from build123d import *

# Parameters (mm, degrees)
SKETCH1_W                                     = 38.1
SKETCH1_H                                     = 44.45
BOSS_EXTRUDE1_DEPTH                           = 5
SKETCH2_W                                     = 38.1
SKETCH2_H                                     = 5
BOSS_EXTRUDE2_DEPTH                           = 25.4
CSK_FOR_8_FLAT_HEAD_SOCKET_CAP_SCREW1_A_COUNT = 2
CSK_FOR_8_FLAT_HEAD_SOCKET_CAP_SCREW1_A_PITCH = 12.7
CSK_FOR_8_FLAT_HEAD_SOCKET_CAP_SCRE_2_COUNT   = 2
CSK_FOR_8_FLAT_HEAD_SOCKET_CAP_SCRE_2_PITCH   = 27.043545921
CSK_FOR_8_FLAT_HEAD_SOCKET_CAP_SCRE_3_COUNT   = 2
CSK_FOR_8_FLAT_HEAD_SOCKET_CAP_SCRE_3_PITCH   = 23.876
CSK_FOR_8_FLAT_HEAD_SOCKET_CAP_SCREW2_A_COUNT = 2
CSK_FOR_8_FLAT_HEAD_SOCKET_CAP_SCREW2_A_PITCH = 19.05
FILLET1_R                                     = 5.08
FILLET2_R                                     = 5.08
FILLET3_R                                     = 1.27


with BuildPart() as part:
    # Sketch1 → Boss-Extrude1 (new body)
    with BuildSketch(Plane.XY):
        with Locations((19.05, 22.225)):
            Rectangle(SKETCH1_W, SKETCH1_H)
    extrude(amount=BOSS_EXTRUDE1_DEPTH)

    # Sketch2 → Boss-Extrude2 (add)
    with BuildSketch(Plane(origin=(0, 0, 0), x_dir=(-1, 0, 0), z_dir=(0, 0, -1))):
        with Locations((-19.05, 2.5)):
            Rectangle(SKETCH2_W, SKETCH2_H)
    extrude(amount=BOSS_EXTRUDE2_DEPTH)

    # Sketch4 → CSK for #8 Flat Head Socket Cap Screw1 (revolve, cut)
    with BuildSketch(Plane(origin=(25.4, 38.1, 0), x_dir=(0, 1, 0), z_dir=(1, 0, 0))):
        Polygon((0, 0), (0, 5), (2.2479, 5), (2.2479, 2.658961536), (4.5593, 0), align=None)
    csk_for_8_flat_head_socket_cap_screw1 = revolve(axis=Axis((25.4, 38.1, -6.35), (0, 0, 1)), mode=Mode.SUBTRACT)

    # CSK for #8 Flat Head Socket Cap Screw1 a: CSK for #8 Flat Head Socket Cap Screw1 ×2
    with Locations(*[(-i * CSK_FOR_8_FLAT_HEAD_SOCKET_CAP_SCREW1_A_PITCH, 0, 0) for i in range(1, CSK_FOR_8_FLAT_HEAD_SOCKET_CAP_SCREW1_A_COUNT)]):
        add(csk_for_8_flat_head_socket_cap_screw1, mode=Mode.SUBTRACT)

    # CSK for _8 Flat Head Socket Cap Scre 2: CSK for #8 Flat Head Socket Cap Screw1 ×2
    with Locations(*[Vector(-0.4696129729783402, -0.8828723891992799, 0) * (i * CSK_FOR_8_FLAT_HEAD_SOCKET_CAP_SCRE_2_PITCH) for i in range(1, CSK_FOR_8_FLAT_HEAD_SOCKET_CAP_SCRE_2_COUNT)]):
        add(csk_for_8_flat_head_socket_cap_screw1, mode=Mode.SUBTRACT)

    # CSK for _8 Flat Head Socket Cap Scre 3: CSK for #8 Flat Head Socket Cap Screw1 ×2
    with Locations(*[(0, -i * CSK_FOR_8_FLAT_HEAD_SOCKET_CAP_SCRE_3_PITCH, 0) for i in range(1, CSK_FOR_8_FLAT_HEAD_SOCKET_CAP_SCRE_3_COUNT)]):
        add(csk_for_8_flat_head_socket_cap_screw1, mode=Mode.SUBTRACT)

    # Sketch6 → CSK for #8 Flat Head Socket Cap Screw2 (revolve, cut)
    with BuildSketch(Plane(origin=(28.575, 5, -12.7), x_dir=(0, 0, 1), z_dir=(1, 0, 0))):
        Polygon((0, 0), (0, 5), (2.2479, 5), (2.2479, 2.658961536), (4.5593, 0), align=None)
    csk_for_8_flat_head_socket_cap_screw2 = revolve(axis=Axis((28.575, 11.35, -12.7), (0, -1, 0)), mode=Mode.SUBTRACT)

    # CSK for #8 Flat Head Socket Cap Screw2 a: CSK for #8 Flat Head Socket Cap Screw2 ×2
    with Locations(*[(-i * CSK_FOR_8_FLAT_HEAD_SOCKET_CAP_SCREW2_A_PITCH, 0, 0) for i in range(1, CSK_FOR_8_FLAT_HEAD_SOCKET_CAP_SCREW2_A_COUNT)]):
        add(csk_for_8_flat_head_socket_cap_screw2, mode=Mode.SUBTRACT)

    # Fillet1
    fillet1_edges = [part.edges().sort_by_distance(p)[0] for p in [
        (19.05, 5, 0),
    ]]
    fillet(fillet1_edges, radius=FILLET1_R)

    # Fillet2
    fillet2_edges = [part.edges().sort_by_distance(p)[0] for p in [
        (19.05, 0, 5),
    ]]
    fillet(fillet2_edges, radius=FILLET2_R)

    # Fillet3
    fillet3_edges = [part.edges().sort_by_distance(p)[0] for p in [
        (38.1, 24.765, 5),
        (38.1, 0, -12.74),
        (38.1, 1.487897552, 3.512102448),
        (0, 0, -12.74),
        (0, 1.487897552, 3.512102448),
        (38.1, 5, -15.24),
        (0, 5, -15.24),
        (38.1, 2.5, -25.4),
        (19.05, 44.45, 5),
        (19.05, 0, -25.4),
        (0, 2.5, -25.4),
        (19.05, 5, -25.4),
        (0, 24.765, 5),
        (19.05, 44.45, 0),
        (0, 27.265, 0),
        (38.1, 27.265, 0),
        (38.1, 6.487897552, -1.487897552),
        (0, 44.45, 2.5),
        (0, 6.487897552, -1.487897552),
        (38.1, 44.45, 2.5),
    ]]
    fillet(fillet3_edges, radius=FILLET3_R)


solid = part.part
Check sheet for the modelled part. Datum: model origin and axes. Units: mm. A direction names the side the tool comes from. Give positions to 0.01 mm unless a question says otherwise; leave off trailing zeros. Write each loop counter-clockwise with the first axis right and the second up, starting at its lowest first coordinate (ties: lowest second). Pieces come first, ordered by that corner, then holes. Notation, with made-up numbers: (2, 68.25) -> (15, 68.25) arc R21 cw to (15, 91.25) -> close; hole circle Ø2 at (-17.5, 76.25). An arc over 180 degrees is marked (long way). One line per item, written item: value. Start each with the question number.
Item 1: Gauge pin test, flat ends, axial feed: pin 1 (10 mm diameter, centred on x = 19.5, y = 28.5, fed in from -Z); pin 2 (4 mm diameter, centred on x = 12.7, y = 38.1, fed in from -Z); pin 3 (5 mm diameter, centred on x = 28.575, z = -12.7, fed in from +Y); pin 4 (15.5 mm diameter, centred on x = 10.5, z = -18, fed in from +Y). Record the tip position at first contact, or that the pin passes through.
Item 2: Draft check along X on faces 6 (the cylindrical face through (14.07, 36.32, 3.81)), 7 (the flat face through (38.1, 13, 2)), 8 (the cylindrical face through (0.382, 44.088, 2.517)). Enter one of: +X half, -X half, draft (parallel to the pull), parting line (faces both ways), or undercut.
Item 3: Section check D-D on y = 22.5. Record the cut outline in (x, z).
Item 4: Section check C-C on x = 3. Record the cut outline in (y, z), then the cut area to 3 significant figures.
Item 5: Section check B-B on z = -12.7. Record the cut outline in (x, y).
Item 6: Section check A-A on y = 38.1. Record the cut outline in (x, z), then the cut area to 3 significant figures.
Item 7: Material ranges on probe 1 along X at (y, z) = (1.3, -12.7); probe 2 along X at (y, z) = (0.6, -12.7); probe 3 along Y at (x, z) = (12, 3), recorded low to high. Write a range as from..to.
Item 8: Tool access check on faces 1 (the cylindrical face through (37.738, 24.397, 4.618)), 2 (the cylindrical face through (0.382, 23.863, 4.638)), 3 (the cylindrical face through (0.382, 26.398, 0.362)), 4 (the flat face through (19, 27, 0)), 5 (the cylindrical face through (37.738, 26.398, 0.382)). Record the directions out of +Z, -Z, +X, -X, +Y, -Y that give a thin tool (end or side, any length) a straight path to the whole face; none if there is none.
Results list:
1. pin 1: z = 0
1. pin 2: through
1. pin 3: y = 2.63
1. pin 4: y = 5
2. face 6: undercut
2. face 7: +X half
2. face 8: -X half
3. outline: (0, 1.27) arc R1.27 ccw to (1.27, 0) -> (36.83, 0) arc R1.27 ccw to (38.1, 1.27) -> (38.1, 3.73) arc R1.27 ccw to (36.83, 5) -> (1.27, 5) arc R1.27 ccw to (0, 3.73) -> close
4. outline: (0, -24.13) arc R1.27 ccw to (1.27, -25.4) -> (3.73, -25.4) arc R1.27 ccw to (5, -24.13) -> (5, -5.08) arc R5.08 cw to (10.08, 0) -> (43.18, 0) arc R1.27 ccw to (44.45, 1.27) -> (44.45, 3.73) arc R1.27 ccw to (43.18, 5) -> (5.08, 5) arc R5.08 ccw to (0, -0.08) -> close
4. area: 348 mm²
5. outline: (0, 1.27) arc R1.27 ccw to (1.27, 0) -> (7.28, 0) -> (7.28, 2.34) -> (4.97, 5) -> (1.27, 5) arc R1.27 ccw to (0, 3.73) -> close; (11.77, 0) -> (26.33, 0) -> (26.33, 2.34) -> (24.02, 5) -> (14.08, 5) -> (11.77, 2.34) -> close; (30.82, 0) -> (36.83, 0) arc R1.27 ccw to (38.1, 1.27) -> (38.1, 3.73) arc R1.27 ccw to (36.83, 5) -> (33.13, 5) -> (30.82, 2.34) -> close
6. outline: (0, 1.27) arc R1.27 ccw to (1.27, 0) -> (8.14, 0) -> (10.45, 2.66) -> (10.45, 5) -> (1.27, 5) arc R1.27 ccw to (0, 3.73) -> close; (14.95, 2.66) -> (17.26, 0) -> (20.84, 0) -> (23.15, 2.66) -> (23.15, 5) -> (14.95, 5) -> close; (27.65, 2.66) -> (29.96, 0) -> (36.83, 0) arc R1.27 ccw to (38.1, 1.27) -> (38.1, 3.73) arc R1.27 ccw to (36.83, 5) -> (27.65, 5) -> close
6. area: 132 mm²
7. probe 1: 0..7.28, 11.77..26.33, 30.82..38.1
7. probe 2: 0.19..7.28, 11.77..26.33, 30.82..37.91
7. probe 3: 1.04..12.09, 16.36..35.96, 40.24..44.45
8. face 1: +Z, +X, +Y, -Y
8. face 2: +Z, -X, +Y, -Y
8. face 3: -Z, -X, +Y
8. face 4: -Z, +X, -X, +Y
8. face 5: -Z, +X, +Y
